```python
from build123d import *

# Parameters (mm, degrees)
SKETCH1_W                                = 50.8
SKETCH1_H                                = 50.8
BOSS_EXTRUDE1_DEPTH                      = 57.15
CUT_EXTRUDE2_START                       = 6.35
SKETCH3_W                                = 38.1
SKETCH3_H                                = 38.1
CUT_EXTRUDE2_DEPTH                       = 44.45
SKETCH5_R                                = 12.7
CUT_EXTRUDE3_DEPTH                       = 6.35
SKETCH6_R                                = 12.7
CUT_EXTRUDE4_DEPTH                       = 6.35
SKETCH7_R                                = 6.35
CUT_EXTRUDE5_DEPTH                       = 6.35
F_3_8_0_375_CLEARANCE_DOWEL_HOLE1_REACH  = 70.392
F_3_8_0_375_CLEARANCE_DOWEL_HOLE1_BORE_R = 6.35
TAP_DRILL_FOR_4_40_TAP1_REACH            = 82.572
TAP_DRILL_FOR_4_40_TAP1_BORE_R           = 1.1303
TAP_START                                = 19.05
TAP_DRILL_FOR_4_40_TAP2_OUTLINE_R        = 1.1303
TAP_DRILL_FOR_4_40_TAP2_DEPTH            = 6.35


# Read off the part's stored shape, not the designer's step: Tap Drill for #4-40 Tap2
with BuildPart() as part:
    # Sketch1 → Boss-Extrude1 (new body)
    with BuildSketch(Plane.XY):
        Rectangle(SKETCH1_W, SKETCH1_H)
    extrude(amount=BOSS_EXTRUDE1_DEPTH)

    # Sketch3 → Cut-Extrude2 (cut)
    with BuildSketch(Plane.XY.offset(CUT_EXTRUDE2_START)):
        Rectangle(SKETCH3_W, SKETCH3_H)
    extrude(amount=CUT_EXTRUDE2_DEPTH, mode=Mode.SUBTRACT)

    # Sketch5 → Cut-Extrude3 (cut)
    with BuildSketch(Plane.ZY.offset(25.4)):
        with Locations(Location((25.4, 0, 0), (0, 0, 270))):
            Circle(SKETCH5_R)
    extrude(amount=-CUT_EXTRUDE3_DEPTH, mode=Mode.SUBTRACT)

    # Sketch6 → Cut-Extrude4 (cut)
    with BuildSketch(Plane(origin=(0, 25.4, 0), x_dir=(1, 0, 0), z_dir=(0, 1, 0))):
        with Locations(Location((0, -38.1, 0), (0, 0, 180))):
            Circle(SKETCH6_R)
    extrude(amount=-CUT_EXTRUDE4_DEPTH, mode=Mode.SUBTRACT)

    # Sketch7 → Cut-Extrude5 (cut)
    with BuildSketch(Plane.XZ.offset(25.4)):
        with Locations((0, 31.75)):
            Circle(SKETCH7_R)
    extrude(amount=-CUT_EXTRUDE5_DEPTH, mode=Mode.SUBTRACT)

    # 3/8 (0.375) Clearance Dowel Hole1 bore (on position points) → 3/8 (0.375) Clearance Dowel Hole1 (cut, up to next)
    with BuildSketch(Plane(origin=(25.4, 0, 38.1), x_dir=(0, 0, 1), z_dir=(1, 0, 0)), mode=Mode.PRIVATE) as f_3_8_0_375_clearance_dowel_hole1_sk1:
        Circle(F_3_8_0_375_CLEARANCE_DOWEL_HOLE1_BORE_R)
    f_3_8_0_375_clearance_dowel_hole1_tool1 = extrude(f_3_8_0_375_clearance_dowel_hole1_sk1.sketch, amount=-F_3_8_0_375_CLEARANCE_DOWEL_HOLE1_REACH, mode=Mode.PRIVATE) & part.part
    add(f_3_8_0_375_clearance_dowel_hole1_tool1.solids().sort_by_distance((25.4, 0, 38.1))[0], mode=Mode.SUBTRACT)

    # Tap Drill for #4-40 Tap1 bore → Tap Drill for #4-40 Tap1 (cut, up to next)
    with BuildSketch(Plane.ZY.offset(25.4), mode=Mode.PRIVATE) as tap_drill_for_4_40_tap1_sk1:
        with Locations((10.4, -15)):
            Circle(TAP_DRILL_FOR_4_40_TAP1_BORE_R)
    tap_drill_for_4_40_tap1_tool1 = extrude(tap_drill_for_4_40_tap1_sk1.sketch, amount=-TAP_DRILL_FOR_4_40_TAP1_REACH, mode=Mode.PRIVATE) & part.part
    # Tap Drill for #4-40 Tap1 bore → Tap Drill for #4-40 Tap1 (cut, up to next)
    with BuildSketch(Plane.ZY.offset(25.4), mode=Mode.PRIVATE) as tap_drill_for_4_40_tap1_sk2:
        with Locations((10.4, 15)):
            Circle(TAP_DRILL_FOR_4_40_TAP1_BORE_R)
    tap_drill_for_4_40_tap1_tool2 = extrude(tap_drill_for_4_40_tap1_sk2.sketch, amount=-TAP_DRILL_FOR_4_40_TAP1_REACH, mode=Mode.PRIVATE) & part.part
    # Tap Drill for #4-40 Tap1 bore → Tap Drill for #4-40 Tap1 (cut, up to next)
    with BuildSketch(Plane.ZY.offset(25.4), mode=Mode.PRIVATE) as tap_drill_for_4_40_tap1_sk3:
        with Locations((40.4, 15)):
            Circle(TAP_DRILL_FOR_4_40_TAP1_BORE_R)
    tap_drill_for_4_40_tap1_tool3 = extrude(tap_drill_for_4_40_tap1_sk3.sketch, amount=-TAP_DRILL_FOR_4_40_TAP1_REACH, mode=Mode.PRIVATE) & part.part
    # Tap Drill for #4-40 Tap1 bore → Tap Drill for #4-40 Tap1 (cut, up to next)
    with BuildSketch(Plane.ZY.offset(25.4), mode=Mode.PRIVATE) as tap_drill_for_4_40_tap1_sk4:
        with Locations((40.4, -15)):
            Circle(TAP_DRILL_FOR_4_40_TAP1_BORE_R)
    tap_drill_for_4_40_tap1_tool4 = extrude(tap_drill_for_4_40_tap1_sk4.sketch, amount=-TAP_DRILL_FOR_4_40_TAP1_REACH, mode=Mode.PRIVATE) & part.part
    add(tap_drill_for_4_40_tap1_tool1.solids().sort_by_distance((-25.4, -15, 10.4))[0], mode=Mode.SUBTRACT)
    add(tap_drill_for_4_40_tap1_tool2.solids().sort_by_distance((-25.4, 15, 10.4))[0], mode=Mode.SUBTRACT)
    add(tap_drill_for_4_40_tap1_tool3.solids().sort_by_distance((-25.4, 15, 40.4))[0], mode=Mode.SUBTRACT)
    add(tap_drill_for_4_40_tap1_tool4.solids().sort_by_distance((-25.4, -15, 40.4))[0], mode=Mode.SUBTRACT)

    # Tap Drill for #4-40 Tap2 outline → Tap Drill for #4-40 Tap2 (cut)
    with BuildSketch(Plane(origin=(0, 0, 0), x_dir=(1, 0, 0), z_dir=(0, 1, 0)).offset(TAP_START)):
        with Locations((-15, -53.1)):
            Circle(TAP_DRILL_FOR_4_40_TAP2_OUTLINE_R)
        with Locations((15, -53.1)):
            Circle(TAP_DRILL_FOR_4_40_TAP2_OUTLINE_R)
        with Locations((15, -23.1)):
            Circle(TAP_DRILL_FOR_4_40_TAP2_OUTLINE_R)
        with Locations((-15, -23.1)):
            Circle(TAP_DRILL_FOR_4_40_TAP2_OUTLINE_R)
    extrude(amount=TAP_DRILL_FOR_4_40_TAP2_DEPTH, mode=Mode.SUBTRACT)


solid = part.part
```
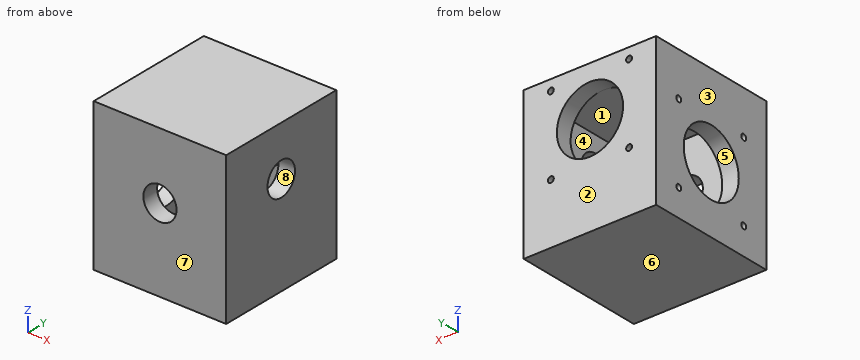
Geometry: final body of the model. Coordinates: model frame, mm. Face numbers are marked on the shaded views. A direction names the side the tool comes from. Coordinates: 2 decimals unless noted, no trailing zeros. Order: outer loops, then holes, each group sorted by start corner. A loop starts at its lowest first (then second) coordinate and runs counter-clockwise, first axis right, second up. Notation, with made-up numbers: M 68.25,-10.5 L 107.25,-10.5 A21 cw 107.25,19.5 Z; hole C 37,76 d8. An arc over 180 degrees is marked long. Answer in a Markdown table with one row per item. Add a question column.
Q1. Reachability of the marked faces 4, 5, 6, 7 and 8 from +Z, -Z, +X, -X, +Y, -Y: full face, straight path, thin tool, end or side. Return the list, or none.
Q2. Mould query, pull axis X, two halves, no side actions, for the marked faces 1, 2 and 3. Classes: released by +X, released by -X, zero draft, split by the parting line, or undercut.
Q3. Line query: L1, parallel to Z at x = -15, y = 23.25; L2, parallel to Y at x = -21.5, z = 10.4; L3, parallel to X at y = -15, z = 13. Output: solid intervals per line, ascending.
Q4. Section query B-B on z = 10.4. Return the cut outline in (x, y), and give its area (3 significant figures).
Q5. Section query D-D on z = 29.5. Return the cut outline in (x, y).
Q6. Contact query for flat-ended pins moving along their axis: P1, Ø1.4, axis at y = 15, z = 40.4, coming from the -X side; P2, Ø19, axis at x = -6, y = -9, coming from the -Z side; P3, Ø15, axis at x = 0, z = 38.1, coming from the +Y side; P4, Ø1.1, axis at x = 15, z = 53, coming from the +Y side. Output: stop coordinate, or through.
Q7. Section query C-C on x = -17.5. Return the cut outline in (y, z), and give its area (3 significant figures).
Q8. Section query A-A on y = 0. Return the cut outline in (x, z).
Completed:
| question | item | result |
|---|---|---|
| 1 | face 4 | none |
| 1 | face 5 | -X |
| 1 | face 6 | -Z, +X, -X, +Y, -Y |
| 1 | face 7 | +Z, -Z, +X, -X, -Y |
| 1 | face 8 | +X |
| 2 | face 1 | undercut |
| 2 | face 2 | zero draft |
| 2 | face 3 | released by -X |
| 3 | L1 | z = 0 to 21.97, 24.23 to 51.97, 54.23 to 57.15 |
| 3 | L2 | y = -25.4 to -16.13, -13.87 to 13.87, 16.13 to 25.4 |
| 3 | L3 | x = -25.4 to -19.05, 19.05 to 25.4 |
| 4 | outline | M -25.4,-25.4 L 25.4,-25.4 L 25.4,25.4 L -25.4,25.4 L -25.4,16.13 L -19.05,16.13 L -19.05,19.05 L 19.05,19.05 L 19.05,-19.05 L -19.05,-19.05 L -19.05,-16.13 L -25.4,-16.13 Z; M -25.4,-13.87 L -19.05,-13.87 L -19.05,13.87 L -25.4,13.87 Z |
| 4 | area | 1,100 mm2 |
| 5 | outline | M -25.4,-25.4 L -5.94,-25.4 L -5.94,-19.05 L -19.05,-19.05 L -19.05,-12.02 L -25.4,-12.02 Z; M -25.4,12.02 L -19.05,12.02 L -19.05,19.05 L -9.35,19.05 L -9.35,25.4 L -25.4,25.4 Z; M 5.94,-25.4 L 25.4,-25.4 L 25.4,25.4 L 9.35,25.4 L 9.35,19.05 L 19.05,19.05 L 19.05,-19.05 L 5.94,-19.05 Z |
| 6 | P1 | stops at x = 19.05 |
| 6 | P2 | stops at z = 0 |
| 6 | P3 | stops at y = -19.05 |
| 6 | P4 | stops at y = 19.05 |
| 7 | outline | M -25.4,0 L 25.4,0 L 25.4,57.15 L -25.4,57.15 Z; hole M -19.05,6.35 L 19.05,6.35 L 19.05,50.8 L -19.05,50.8 Z |
| 7 | area | 1,210 mm2 |
| 8 | outline | M -25.4,0 L 25.4,0 L 25.4,31.75 L 19.05,31.75 L 19.05,6.35 L -19.05,6.35 L -19.05,12.7 L -25.4,12.7 Z; M -25.4,38.1 L -19.05,38.1 L -19.05,50.8 L 19.05,50.8 L 19.05,44.45 L 25.4,44.45 L 25.4,57.15 L -25.4,57.15 Z |
